For this review, take the finished solid that the model builds, in its own axes (mm). Coordinates: 2 decimals unless noted, no trailing zeros. Loops run counter-clockwise (first coordinate to the right, second up) from the corner with the lowest first, then second, coordinate; pieces in that order, holes last. Notation, with made-up numbers: (-26.5, -6.5) -> (4.5, -6.5) arc R30 cw to (4.5, 16.5) -> close; hole circle Ø4 at (36.5, -1). An arc over 180 degrees is marked (long way). Answer in a Markdown table with one row per item.
from build123d import *

# Parameters (mm, degrees)
F0_R     = 1.85
F1_DEPTH = 4.826


with BuildPart() as f1:
    # F0 (on Top) → F1 (new body)
    with BuildSketch(Plane.XY):
        with BuildLine():
            Line((0, 50.8), (-6.35, 50.8))
            ThreePointArc((-6.35, 50.8), (-10.840128, 48.940128), (-12.7, 44.45))
            Line((-12.7, 44.45), (-12.7, -50.8))
            add(Edge.make_bspline(
                [(0, 50.8), (-12.7, 50.8), (-12.7, -12.351775), (-12.7, -50.8)],
                knots=[0, 0, 0, 0, 102.390673, 102.390673, 102.390673, 102.390673], degree=3))
        make_face()
        with BuildLine():
            add(Edge.make_bspline(
                [(0, 50.8), (12.7, 50.8), (12.7, -12.351775), (12.7, -50.8)],
                knots=[0, 0, 0, 0, 102.390673, 102.390673, 102.390673, 102.390673], degree=3))
            add(Edge.make_bspline(
                [(0, 50.8), (-12.7, 50.8), (-12.7, -12.351775), (-12.7, -50.8)],
                knots=[0, 0, 0, 0, 102.390673, 102.390673, 102.390673, 102.390673], degree=3))
            Line((-12.7, -50.8), (12.7, -50.8))
        make_face()
        with Locations((-8, -39.8)):
            Circle(F0_R, mode=Mode.SUBTRACT)
        with Locations((8, -39.8)):
            Circle(F0_R, mode=Mode.SUBTRACT)
        with BuildLine():
            Line((6.35, 50.8), (0, 50.8))
            add(Edge.make_bspline(
                [(0, 50.8), (12.7, 50.8), (12.7, -12.351775), (12.7, -50.8)],
                knots=[0, 0, 0, 0, 102.390673, 102.390673, 102.390673, 102.390673], degree=3))
            Line((12.7, -50.8), (12.7, 44.45))
            ThreePointArc((12.7, 44.45), (10.840128, 48.940128), (6.35, 50.8))
        make_face()
    extrude(amount=F1_DEPTH)


solid = f1.part
Item 1: Take a section at B-B, the plane z = 1.5. State the section outline as (x, y) points.
Worked answers:
| item | result |
|---|---|
| outline | (-12.7, -50.8) -> (12.7, -50.8) -> (12.7, 44.45) arc R6.35 ccw to (6.35, 50.8) -> (-6.35, 50.8) arc R6.35 ccw to (-12.7, 44.45) -> close; hole circle Ø3.7 at (-8, -39.8); hole circle Ø3.7 at (8, -39.8) |
Item 2: The part is to be moulded in two halves that separate along Y. For faces 1 (the flat face through (0, 1, 0)), 2 (the cylindrical face through (-8.401, -41.606, 2.379)), 3 (the cylindrical face through (7.599, -41.606, 2.379)), 4 (the cylindrical face through (-10.79, 48.99, 2.38)), say which applies: +Y half, -Y half, draft (parallel to the pull), parting line (faces both ways), or undercut.
Worked answers:
| item | result |
|---|---|
| face 1 | draft |
| face 2 | undercut |
| face 3 | undercut |
| face 4 | +Y half |
Item 3: For L1, parallel to X at y = -40, z = 3; L2, parallel to Y at x = -8, z = 3.7; L3, parallel to Y at x = 10.25, z = 4.5, list the stretches that pass through material, from the lowest coordinate up.
Worked answers:
| item | result |
|---|---|
| L1 | -12.7 to -9.84, -6.16 to 6.16, 9.84 to 12.7 |
| L2 | -50.8 to -41.65, -37.95 to 50.58 |
| L3 | -50.8 to 49.46 |
Item 4: Take a section at C-C, the plane x = -8.25. State the section outline as (y, z) points.
Worked answers:
| item | result |
|---|---|
| outline | (-50.8, 0) -> (-41.63, 0) -> (-41.63, 4.83) -> (-50.8, 4.83) -> close; (-37.97, 0) -> (50.51, 0) -> (50.51, 4.83) -> (-37.97, 4.83) -> close |
Item 5: Take a section at A-A, the plane y = -39.8. State the section outline as (x, z) points, and give its area (3 significant figures).
Worked answers:
| item | result |
|---|---|
| outline | (-12.7, 0) -> (-9.85, 0) -> (-9.85, 4.83) -> (-12.7, 4.83) -> close; (-6.15, 0) -> (6.15, 0) -> (6.15, 4.83) -> (-6.15, 4.83) -> close; (9.85, 0) -> (12.7, 0) -> (12.7, 4.83) -> (9.85, 4.83) -> close |
| area | 86.9 mm² |
